from build123d import *

# Parameters (mm, degrees)
EXTRUDE_1_DEPTH     = 12
SKETCH_2_W          = 32
SKETCH_2_H          = 3
EXTRUDE_2_DEPTH     = 25
SKETCH_3_R          = 3.25
CUT_EXTRUDE_1_DEPTH = 38
SKETCH_4_R          = 2.271913659
EXTRUDE_3_DEPTH     = 10
CHAMFER_2_SIZE      = 2
CHAMFER_3_SIZE      = 2
EXTRUDE_4_DEPTH     = 4
CHAMFER_4_SIZE      = 2
SKETCH_6_R          = 1.8
CUT_EXTRUDE_2_DEPTH = 8
EXTRUDE_5_DEPTH     = 0.8
SKETCH_8_R          = 2.271913659
CUT_EXTRUDE_3_DEPTH = 23


with BuildPart() as part:
    # 草图1 → 凸台-拉伸1 (new body)
    with BuildSketch(Plane.XY):
        Polygon((16, 0), (-16, 0), (-16, 18), (-6, 18), (-6, 5), (6, 5), (6, 18), (16, 18), align=None)
    extrude(amount=EXTRUDE_1_DEPTH)

    # 草图2 → 凸台-拉伸2 (add)
    with BuildSketch(Plane.XY.offset(12)):
        with Locations((0, 1.5)):
            Rectangle(SKETCH_2_W, SKETCH_2_H)
    extrude(amount=EXTRUDE_2_DEPTH)

    # 草图3 → 切除-拉伸1 (cut)
    with BuildSketch(Plane.ZY.offset(16)):
        with Locations((6, 13.5)):
            Circle(SKETCH_3_R)
    extrude(amount=-CUT_EXTRUDE_1_DEPTH, mode=Mode.SUBTRACT)

    # 草图4 → 凸台-拉伸3 (add)
    with BuildSketch(Plane.ZY.offset(16)):
        Polygon((2.061755591, 18), (12.158971032, 38.730393582), (22.947301651, 33.47568879), (12, 11), (12, 18), align=None)
        with Locations((16, 30.820508076)):
            Circle(SKETCH_4_R, mode=Mode.SUBTRACT)
    extrude_3 = extrude(amount=-EXTRUDE_3_DEPTH)

    # 镜向1: 凸台-拉伸3 across plane
    add(extrude_3.mirror(Plane(origin=(0, 0, 0), x_dir=(0, 0, 1), z_dir=(1, 0, 0))))

    # 倒角2
    chamfer_2_edges = [part.edges().sort_by_distance(p)[0] for p in [
        (11, 18, 0),
        (-11, 18, 0),
    ]]
    chamfer(chamfer_2_edges, length=CHAMFER_2_SIZE)

    # 倒角3
    chamfer_3_edges = [part.edges().sort_by_distance(p)[0] for p in [
        (-11, 38.730393582, 12.158971032),
        (-11, 33.47568879, 22.947301651),
        (11, 33.47568879, 22.947301651),
        (11, 38.730393582, 12.158971032),
    ]]
    chamfer(chamfer_3_edges, length=CHAMFER_3_SIZE)

    # 草图5 → 凸台-拉伸4 (add)
    with BuildSketch(Plane.ZY.offset(16)):
        Polygon((15.409511151, 18), (26, 3), (12, 3), (12, 11), align=None)
    extrude_4 = extrude(amount=-EXTRUDE_4_DEPTH)

    # 镜向2: 凸台-拉伸4 across plane
    add(extrude_4.mirror(Plane(origin=(0, 0, 0), x_dir=(0, 0, 1), z_dir=(1, 0, 0))))

    # 倒角4
    chamfer_4_edges = [part.edges().sort_by_distance(p)[0] for p in [
        (0, 0, 0),
    ]]
    chamfer(chamfer_4_edges, length=CHAMFER_4_SIZE)

    # 草图6 → 切除-拉伸2 (cut)
    with BuildSketch(Plane(origin=(0, 3, 0), x_dir=(1, 0, 0), z_dir=(0, 1, 0))):
        with Locations(Location((0, -32.750411326, 0), (0, 0, 270))):
            Circle(SKETCH_6_R)
        with Locations(Location((-9, -32.750411326, 0), (0, 0, 270))):
            Circle(SKETCH_6_R)
        with Locations(Location((9, -32.750411326, 0), (0, 0, 180))):
            Circle(SKETCH_6_R)
    extrude(amount=-CUT_EXTRUDE_2_DEPTH, mode=Mode.SUBTRACT)

    # 草图7 → 凸台-拉伸5 (add)
    with BuildSketch(Plane.ZY.offset(-6)):
        Polygon((11.2831869, 36.932338479), (13.957026135, 37.85460945), (21.149246548, 34.351472922), (22.071517519, 31.677633686), (19.006273057, 25.384440825), (16.525669772, 24.528821546), (9.073561717, 28.158542333), (8.217942438, 30.639145618), align=None)
    extrude_5 = extrude(amount=EXTRUDE_5_DEPTH)

    # 镜向3: 凸台-拉伸5 across plane
    add(extrude_5.mirror(Plane(origin=(0, 0, 0), x_dir=(0, 0, 1), z_dir=(1, 0, 0))))

    # 草图8 → 切除-拉伸3 (cut)
    with BuildSketch(Plane.ZY.offset(6)):
        with Locations((16, 30.820508076)):
            Circle(SKETCH_8_R)
    extrude(amount=-CUT_EXTRUDE_3_DEPTH, mode=Mode.SUBTRACT)


solid = part.part
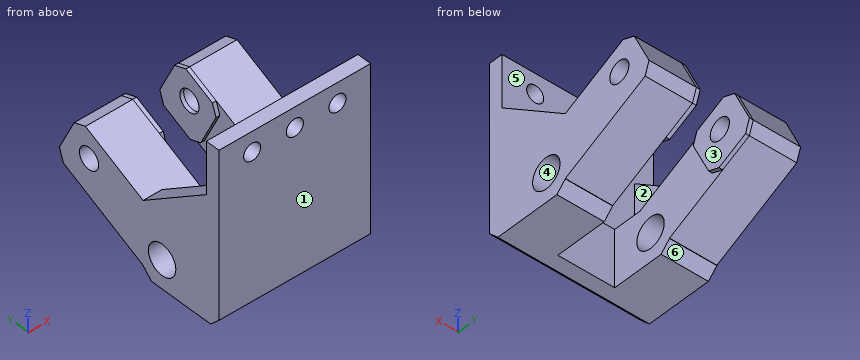
The listing builds one solid part. Answer for the finished solid, in the listing's coordinates (mm). Face numbers are marked on the shaded views. A direction names the side the tool comes from. Round coordinates to 2 decimals unless told otherwise and drop trailing zeros. Write each loop counter-clockwise with the first axis right and the second up, starting at its lowest first coordinate (ties: lowest second). Pieces come first, ordered by that corner, then holes. Notation, with made-up numbers: M 89,-7.75 L 107,-7.75 A28 ccw 107,12.25 Z; hole C 65,29.25 d4. An arc over 180 degrees is marked long. Write each question's results on one line, items separated by ' | '. Start each with the question number.
Item 1: A cutting plane is placed at C-C on z = 7. Write down the section's boundary in (x, y).
Item 2: A cutting plane is placed at B-B on y = 13.5. Write down the section's boundary in (x, z), and give its area (3 significant figures).
Item 3: Straight lines are drawn through the part: L1, parallel to X at y = 15.5, z = 12.5; L2, parallel to Y at x = -10, z = 14; L3, parallel to Y at x = -9, z = 16. For each, find the intervals that lie inside material, in ascending order. Write a range as [from, to].
Item 4: Flat-ended cylindrical pins translate along their axes: pin 1 Ø8 at (y, z) = (21.5, 24.5) entering from -X; pin 2 Ø2 at (x, y) = (-9, 23.5) entering from -Z; pin 3 Ø4 at (x, y) = (-8.5, 28) entering from +Z; pin 4 Ø8 at (x, y) = (-12, 21) entering from +Z. Find the tip coordinate at first contact, or state that the pin passes through.
Item 5: For the marked faces 1, 2 and 3, determine the directions among +Z, -Z, +X, -X, +Y, -Y from which every point of the face is accessible in a straight line to the end or side of a thin tool.
Item 6: A cutting plane is placed at D-D on y = 17.5. Write down the section's boundary in (x, z).
Item 7: For a pull along Z with two mould halves and no side action, classify the marked faces 4, 5 and 6 as pulls with the +Z half, pulls with the -Z half, needs draft (parallel to the pull), parting line crosses it, or undercut.
Item 8: A cutting plane is placed at A-A on x = -10. Write down the section's boundary in (y, z).
Check sheet entries:
1) outline: M -16,0 L 16,0 L 16,10.41 L 6,10.41 L 6,5 L -6,5 L -6,10.41 L -16,10.41 Z; M -16,16.59 L -6,16.59 L -6,28.14 L -16,28.14 Z; M 6,16.59 L 16,16.59 L 16,28.14 L 6,28.14 Z
2) outline: M -16,0 L -6,0 L -6,2.75 L -16,2.75 Z; M -16,9.25 L -6,9.25 L -6,13.22 L -12,13.22 L -12,18.59 L -16,18.59 Z; M 6,0 L 16,0 L 16,2.75 L 6,2.75 Z; M 6,9.25 L 16,9.25 L 16,18.59 L 12,18.59 L 12,13.22 L 6,13.22 Z | area: 177 mm²
3) L1: [-16, -6], [6, 16] | L2: [0, 3], [15.11, 29.74], [31.9, 37.83] | L3: [0, 3], [19.21, 28.55], [33.09, 36.86]
4) pin 1: through | pin 2: z = 4.25 | pin 3: z = 21.25 | pin 4: z = 18.82
5) face 1: +Z, -Z, +X, -X, -Y | face 2: +Z | face 3: +Z, -Z, +Y
6) outline: M -16,1.5 L -6,1.5 L -6,15.17 L -12,15.17 L -12,15.76 L -16,15.76 Z; M 6,1.5 L 16,1.5 L 16,15.76 L 12,15.76 L 12,15.17 L 6,15.17 Z
7) face 4: undercut | face 5: needs draft | face 6: pulls with the -Z half
8) outline: M 0,2 L 2,0 L 16,0 L 18,2 L 18,2.06 L 36.93,11.28 L 37.85,13.96 L 34.35,21.15 L 31.68,22.07 L 11,12 L 3,12 L 3,31.25 L 0,31.25 Z; M 0,34.25 L 3,34.25 L 3,37 L 0,37 Z; hole C 13.5,6 d6.5; hole C 30.82,16 d4.54
